Input: dimensioned drawing with shaded views. Units: mm. Origin: part minimum x, y, z. Coordinates: 2 decimals unless noted, no trailing zeros. Loops run counter-clockwise (first coordinate to the right, second up) from the corner with the lowest first, then second, coordinate; pieces in that order, holes last. Notation, with made-up numbers: (56.25, 12) -> (102.25, 12) arc R21 cw to (102.25, 22) -> close; hole circle Ø9 at (-29.75, 78.5). An arc over 180 degrees is marked (long way). Answer as CSV lines item,"result".
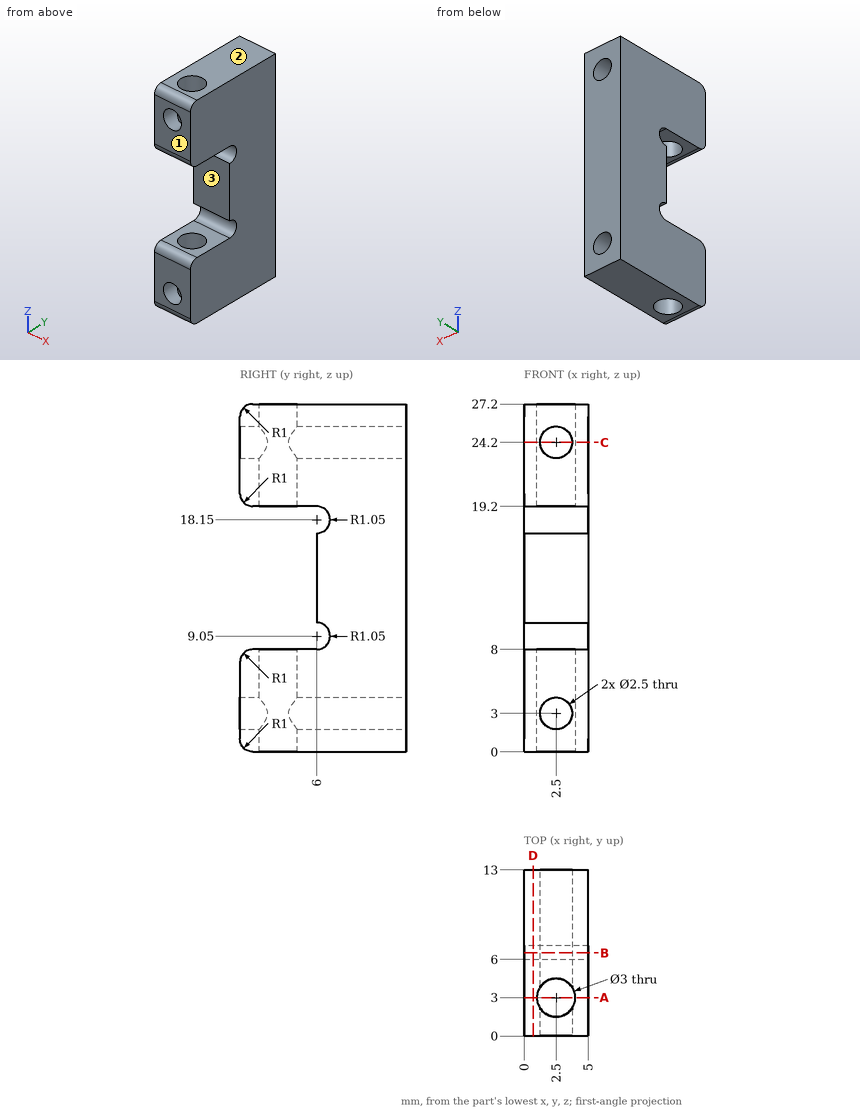
(1) Cut plane C-C (z = 24.2). Return the cut outline in (x, y), then the cut area to 3 significant figures.
Computed values:
outline,"(0, 0) -> (1.25, 0) -> (1.25, 2.17) arc R1.5 cw to (1.25, 3.83) -> (1.25, 13) -> (0, 13) -> close; (3.75, 0) -> (5, 0) -> (5, 13) -> (3.75, 13) -> (3.75, 3.83) arc R1.5 cw to (3.75, 2.17) -> close"
area,"31.9 mm^2"
(2) Material intervals for L1, parallel to Z at x = 2.5, y = 1.4; L2, parallel to Z at x = 2.5, y = 10; L3, parallel to Y at x = 2.5, z = 4.75, sorted ascending. Write a range as [from, to].
Computed values:
L1,"[0, 1.75], [4.25, 8], [19.2, 22.95], [25.45, 27.2]"
L2,"[0, 1.75], [4.25, 22.95], [25.45, 27.2]"
L3,"[0, 1.5], [4.5, 13]"
(3) Cut plane B-B (y = 6.5). Return the cut outline in (x, z).
Computed values:
outline,"(0, 0) -> (5, 0) -> (5, 8.13) -> (0, 8.13) -> close; (0, 9.97) -> (5, 9.97) -> (5, 17.23) -> (0, 17.23) -> close; (0, 19.07) -> (5, 19.07) -> (5, 27.2) -> (0, 27.2) -> close; hole circle Ø2.5 at (2.5, 3); hole circle Ø2.5 at (2.5, 24.2)"
(4) Pin query (flat end, axial travel): pin 1 Ø2 at (x, z) = (2.5, 24.2) entering from -Y; pin 2 Ø1.5 at (x, z) = (4, 17) entering from -Y. Return the tip coordinate at first contact, or that it passes through.
Computed values:
pin 1,"through"
pin 2,"y = 6"
(5) Draft query along Z for the marked faces 1, 2 and 3. Return one class per face: released by +Z, released by -Z, zero draft, split by the parting line, or undercut.
Computed values:
face 1,"zero draft"
face 2,"released by +Z"
face 3,"undercut"
(6) Cut plane A-A (y = 3). Return the cut outline in (x, z), then the cut area to 3 significant figures.
Computed values:
outline,"(0, 0) -> (1, 0) -> (1, 8) -> (0, 8) -> close; (0, 19.2) -> (1, 19.2) -> (1, 27.2) -> (0, 27.2) -> close; (4, 0) -> (5, 0) -> (5, 8) -> (4, 8) -> close; (4, 19.2) -> (5, 19.2) -> (5, 27.2) -> (4, 27.2) -> close"
area,"32.0 mm^2"
(7) Cut plane D-D (x = 0.7). Return the cut outline in (y, z).
Computed values:
outline,"(0, 1) arc R1 ccw to (1, 0) -> (13, 0) -> (13, 27.2) -> (1, 27.2) arc R1 ccw to (0, 26.2) -> (0, 20.2) arc R1 ccw to (1, 19.2) -> (6, 19.2) arc R1.05 cw to (6, 17.1) -> (6, 10.1) arc R1.05 cw to (6, 8) -> (1, 8) arc R1 ccw to (0, 7) -> close"
